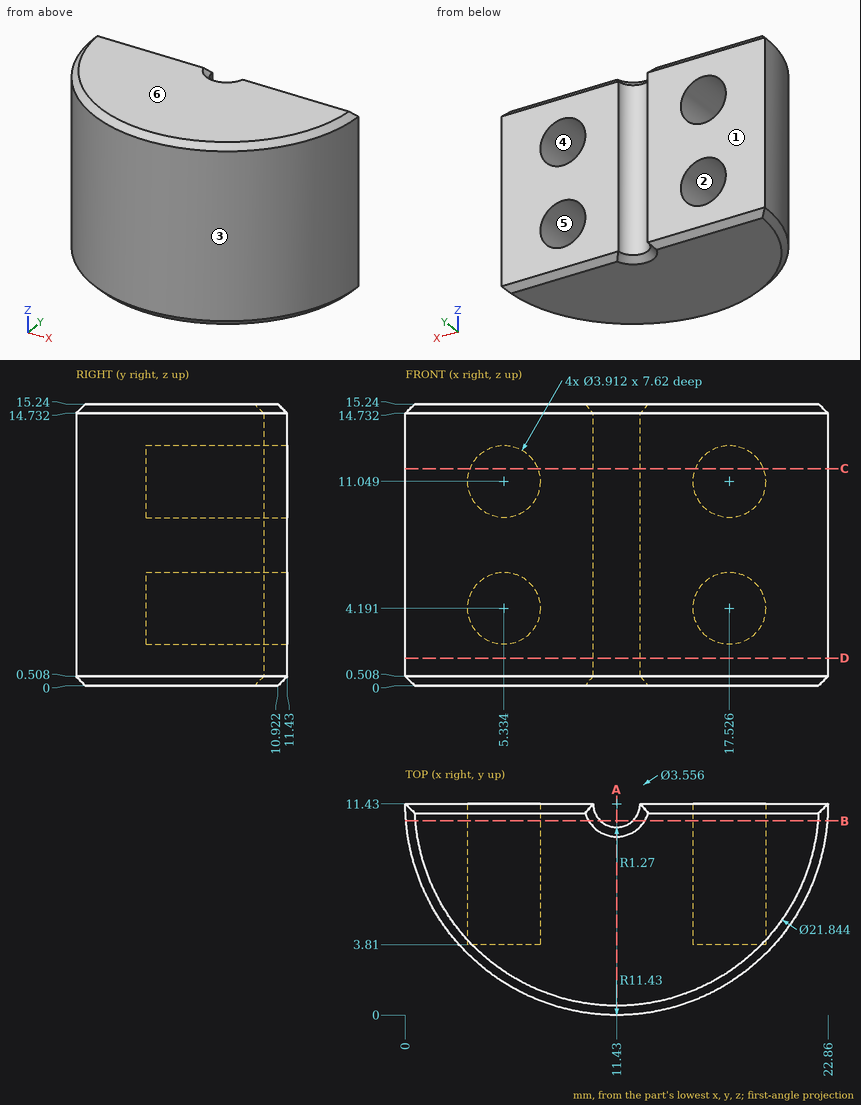
Here's the drawing with two shaded views (mm, measured from the low corner). I have some questions. A direction names the side the tool comes from. Give positions to 0.01 mm unless a question says otherwise; leave off trailing zeros. Write each loop counter-clockwise with the first axis right and the second up, starting at its lowest first coordinate (ties: lowest second). Pieces come first, ordered by that corner, then holes. Notation, with made-up numbers: (19, -38.5) -> (62, -38.5) arc R10 cw to (62, -25.5) -> close; hole circle Ø8 at (-33, 13). An arc over 180 degrees is marked (long way). Use one line per item in the form item = value. Start each with the question number.
1. Imagine slicing it at A-A on x = 11.43. List the corners of the cut face in (y, z) for me.
2. Imagine slicing it at D-D on z = 1.5. List the corners of the cut face in (x, y) for me.
3. If I drill on L1, parallel to X at y = 4.75, z = 4 (1 decimal); L2, parallel to X at y = 9, z = 3.25; L3, parallel to Z at x = 17.75, y = 9, over which ranges is the centre line in solid material (lowest first)?
4. On a 3-axis mill with a long thin cutter (end or side, diameter ignored), from which of +Z, -Z, +X, -X, +Y, -Y can I reach the whole of each face in a straight line? I mean the marked faces 1 and 2. Say none if no direction works.
5. Imagine slicing it at B-B on y = 10.5. State how many separate pieces and enclosed holes the cut face has.
6. Will these pins go through, and if not, where does the flat tip stop? pin 1 Ø2.5 at (x, z) = (5.334, 11.049) entering from +Y; pin 2 Ø3 at (y, z) = (6.5, 13.5) entering from -X; pin 3 Ø1.5 at (x, z) = (9, 8.5) entering from -Y; pin 4 Ø3 at (x, y) = (19, 2) entering from +Z.
7. Thinking about a two-plate mould opening in Z: for the marked faces 3, 4, 5 and 6, which applies, +Z half, -Z half, draft (parallel to the pull), parting line (faces both ways), or undercut?
8. Imagine slicing it at C-C on z = 11.75. List the corners of the cut face in (x, y) for me.
Entries:
q1.outline = (0, 0.51) -> (0.51, 0) -> (9.65, 0) -> (10.16, 0.51) -> (10.16, 14.73) -> (9.65, 15.24) -> (0.51, 15.24) -> (0, 14.73) -> close
q2.outline = (0, 11.43) arc R11.43 ccw to (22.86, 11.43) -> (12.7, 11.43) arc R1.27 cw to (10.16, 11.43) -> close
q3.L1 = 2.2 to 3.4, 7.3 to 15.6, 19.5 to 20.7
q3.L2 = 0.26 to 3.62, 7.05 to 15.81, 19.24 to 22.6
q3.L3 = 0 to 2.25, 6.13 to 9.11, 12.99 to 15.24
q4.face_1 = +Z, -Z, +X, -X, +Y
q4.face_2 = +Y
q5.separate_pieces = 2
q5.enclosed_holes = 4
q6.pin_1 = 3.81
q6.pin_2 = 0.53
q6.pin_3 = 0.12
q6.pin_4 = 15.24
q7.face_3 = draft
q7.face_4 = undercut
q7.face_5 = undercut
q7.face_6 = +Z half
q8.outline = (0, 11.43) arc R11.43 ccw to (22.86, 11.43) -> (19.35, 11.43) -> (19.35, 3.81) -> (15.7, 3.81) -> (15.7, 11.43) -> (12.7, 11.43) arc R1.27 cw to (10.16, 11.43) -> (7.16, 11.43) -> (7.16, 3.81) -> (3.51, 3.81) -> (3.51, 11.43) -> close
